from build123d import *

# Parameters (mm, degrees)
SKETCH_1_W          = 36
SKETCH_1_H          = 16
EXTRUDE_1_DEPTH     = 80
SKETCH_3_W          = 24
SKETCH_3_H          = 74
CUT_EXTRUDE_1_DEPTH = 84.546394297
FILLET_1_R          = 5
FILLET_2_R          = 2
SKETCH_4_R          = 3
CUT_EXTRUDE_2_DEPTH = 89.090862182
SKETCH_2_R          = 3.3
CUT_EXTRUDE_3_DEPTH = 83.389319696
SKETCH_5_W          = 2.5
SKETCH_5_H          = 8
CUT_EXTRUDE_4_DEPTH = 20
SKETCH_6_R          = 1.6
CUT_EXTRUDE_5_DEPTH = 88.099081511


with BuildPart() as part:
    # 草图1 → 凸台-拉伸1 (new body)
    with BuildSketch(Plane(origin=(0, 0, 0), x_dir=(1, 0, 0), z_dir=(0, 1, 0))):
        Rectangle(SKETCH_1_W, SKETCH_1_H)
    extrude(amount=-EXTRUDE_1_DEPTH)

    # 草图3 → 切除-拉伸1 (cut, through all)
    with BuildSketch(Plane.XY.offset(8)):
        with Locations((0, -43)):
            Rectangle(SKETCH_3_W, SKETCH_3_H)
    extrude(amount=-CUT_EXTRUDE_1_DEPTH, mode=Mode.SUBTRACT)

    # 圆角1
    fillet_1_edges = [part.edges().sort_by_distance(p)[0] for p in [
        (15, -80, -8),
        (-15, -80, -8),
        (15, -80, 8),
        (-12, -6, 0),
        (12, -6, 0),
        (18, 0, 0),
        (-18, 0, 0),
        (-15, -80, 8),
    ]]
    fillet(fillet_1_edges, radius=FILLET_1_R)

    # 圆角2
    fillet_2_edges = [part.edges().sort_by_distance(p)[0] for p in [
        (-12, -43, -8),
        (-18, -40, -8),
        (0, 0, -8),
        (18, -40, -8),
        (12, -43, -8),
        (0, -6, -8),
        (16.535533906, -1.464466094, -8),
        (-16.535533906, -1.464466094, -8),
        (-18, -80, 0),
        (-18, -40, 8),
        (-18, -78.535533906, 6.535533906),
        (-18, -78.535533906, -6.535533906),
        (-12, -80, 0),
        (-12, -43, 8),
        (-12, -78.535533906, 6.535533906),
        (-12, -78.535533906, -6.535533906),
        (12, -43, 8),
        (12, -80, 0),
        (12, -78.535533906, 6.535533906),
        (12, -78.535533906, -6.535533906),
        (18, -80, 0),
        (18, -40, 8),
        (18, -78.535533906, 6.535533906),
        (18, -78.535533906, -6.535533906),
        (0, -6, 8),
        (0, 0, 8),
        (16.535533906, -1.464466094, 8),
        (-16.535533906, -1.464466094, 8),
        (10.535533906, -7.464466094, 8),
        (10.535533906, -7.464466094, -8),
        (-10.535533906, -7.464466094, 8),
        (-10.535533906, -7.464466094, -8),
    ]]
    fillet(fillet_2_edges, radius=FILLET_2_R)

    # 草图4 → 切除-拉伸2 (cut, through all)
    with BuildSketch(Plane(origin=(18, 0, 0), x_dir=(0, 0, -1), z_dir=(1, 0, 0))):
        with Locations((0, -72)):
            Circle(SKETCH_4_R)
    extrude(amount=-CUT_EXTRUDE_2_DEPTH, mode=Mode.SUBTRACT)

    # 草图2 → 切除-拉伸3 (cut, through all)
    with BuildSketch(Plane(origin=(0, 0, 0), x_dir=(1, 0, 0), z_dir=(0, 1, 0))):
        with Locations(Location((0, 0, 0), (0, 0, 270))):
            Circle(SKETCH_2_R)
    extrude(amount=-CUT_EXTRUDE_3_DEPTH, mode=Mode.SUBTRACT)

    # 草图5 → 切除-拉伸4 (cut)
    with BuildSketch(Plane(origin=(0, 0, 0), x_dir=(1, 0, 0), z_dir=(0, 1, 0))):
        with Locations((-16.75, 0)):
            Rectangle(SKETCH_5_W, SKETCH_5_H)
        with Locations((16.75, 0)):
            Rectangle(SKETCH_5_W, SKETCH_5_H)
    extrude(amount=-CUT_EXTRUDE_4_DEPTH, mode=Mode.SUBTRACT)

    # 草图6 → 切除-拉伸5 (cut, through all)
    with BuildSketch(Plane.ZY.offset(15.5)):
        with Locations((0, -15)):
            Circle(SKETCH_6_R)
    extrude(amount=-CUT_EXTRUDE_5_DEPTH, mode=Mode.SUBTRACT)


solid = part.part
Build history of the part. All positions in model axes, mm. A direction names the side the tool comes from. Give positions to 0.01 mm unless a question says otherwise; leave off trailing zeros. Order: outer loops, then holes, each group sorted by start corner. A loop starts at its lowest first (then second) coordinate and runs counter-clockwise, first axis right, second up. Notation, with made-up numbers: M -23,86.5 L 17,86.5 A26 cw 17,125.5 Z; hole C 52,-19.5 d7. An arc over 180 degrees is marked long. Put each result on its own line as item: value.
Item 1: Two-plate mould, pull along X, no slides. Class faces 1 (the cylindrical face through (-17.43, -40.49, -7.4)), 2 (the cylindrical face through (-12.6, -43.45, 7.43)), 3 (the flat face through (-14.3, -32.9, -8)): +X half, -X half, draft (parallel to the pull), parting line (faces both ways), or undercut.
From the geometry:
face 1: -X half
face 2: undercut
face 3: draft
Item 2: Slice it at A-A, the plane y = -52. Write the cut outline in (x, z).
From the geometry:
outline: M -18,-6 A2 ccw -16,-8 L -14,-8 A2 ccw -12,-6 L -12,6 A2 ccw -14,8 L -16,8 A2 ccw -18,6 Z; M 12,-6 A2 ccw 14,-8 L 16,-8 A2 ccw 18,-6 L 18,6 A2 ccw 16,8 L 14,8 A2 ccw 12,6 Z
Item 3: Probe line 1 (X direction, y = -73.5, z = -5.5); line 2 (X direction, y = -18.5, z = 0.75); line 3 (Y direction, x = -12.95, z = 0). List the from-to ranges inside material, lowest first. Write a range as [from, to].
From the geometry:
line 1: x = [-18, -12], [12, 18]
line 2: x = [-15.5, -12], [12, 15.5]
line 3: y = [-79.7, -75], [-69, -16.6], [-13.4, 0]
Item 4: Slice it at B-B, the plane y = -15. Give the number of separate pieces and of enclosed holes in the cut face, plus the area to 3 significant figures.
From the geometry:
separate pieces: 4
enclosed holes: 0
area: 123 mm2
Item 5: Flat gauge pins, fed straight in: pin 1 Ø3.5 at (y, z) = (-15, 0) entering from -X; pin 2 Ø0.8 at (x, z) = (17, 0) entering from +Y; pin 3 Ø6 at (x, z) = (-2, 0.5) entering from -Y; pin 4 Ø8.5 at (x, z) = (0, 0) entering from +Y. Where does each tip first touch, or does it go through?
From the geometry:
pin 1: stops at x = -15.5
pin 2: stops at y = -20
pin 3: stops at y = -6
pin 4: stops at y = 0
Item 6: 3-axis set-ups, long thin cutter, end or side, ignore diameter. For faces 4 (the flat face through (-17, -10, 4)), 5 (the cylindrical face through (-12.6, -42.55, -7.43)), 6 (the flat face through (17, -20, 0)), 7 (the cylindrical face through (11, -8, 0)): which of +Z, -Z, +X, -X, +Y, -Y reach the whole face in a straight line?
From the geometry:
face 4: -X, +Y
face 5: -Z, -Y
face 6: +X, +Y
face 7: +Z, -Z, -Y
Item 7: Slice it at C-C, the plane x = 0. Write the cut outline in (y, z).
From the geometry:
outline: M -6,-6 A2 ccw -4,-8 L -2,-8 A2 ccw 0,-6 L 0,-3.3 L -6,-3.3 Z; M -6,3.3 L 0,3.3 L 0,6 A2 ccw -2,8 L -4,8 A2 ccw -6,6 Z
